Study the drawing (mm; zero at the part's minimum x, y, z) and answer. A direction names the side the tool comes from. Coordinates: 2 decimals unless noted, no trailing zeros. Loops run counter-clockwise (first coordinate to the right, second up) from the corner with the lowest first, then second, coordinate; pieces in that order, holes last. Notation, with made-up numbers: (51, 42.5) -> (70, 42.5) arc R25 cw to (70, 57.5) -> close; hole circle Ø2 at (16, -21). An arc over 180 degrees is marked (long way). Answer as a JSON object with one key per item and string values. Group by question number.
Q1. The part is cut by section A-A on x = 27.5. Write down the section's boundary in (y, z), and give its area (3 significant figures).
Q2. For the marked faces 1, 2 and 3, determine the directions among +Z, -Z, +X, -X, +Y, -Y from which every point of the face is accessible in a straight line to the end or side of a thin tool.
Q3. Each of these flat-tipped pins is pushed along its axis until it touches: P1, Ø1, axis at y = 12.5, z = 3.5, coming from the -X side; P2, Ø13, axis at x = 7, y = 17, coming from the -Z side; P3, Ø1, axis at x = 17, y = 24.5, coming from the +Z side. Where does it stop, or does it pass through?
Q4. Determine the mould class of the marked faces 4, 5 and 6 for opening direction X: released by +X, released by -X, zero draft, split by the parting line, or undercut.
Q5. The part is cut by section B-B on y = 11.5. State how many separate pieces and enclosed holes the cut face has, and give its area (3 significant figures).
Q6. Straight lines are drawn through the part: line 1 along X through (y, z) = (11.4, 2.5); line 2 along Y through (x, z) = (15.25, 2); line 3 along X through (y, z) = (11.75, 3.3). For each, find the intervals that lie inside material, in ascending order. Write a range as [from, to].
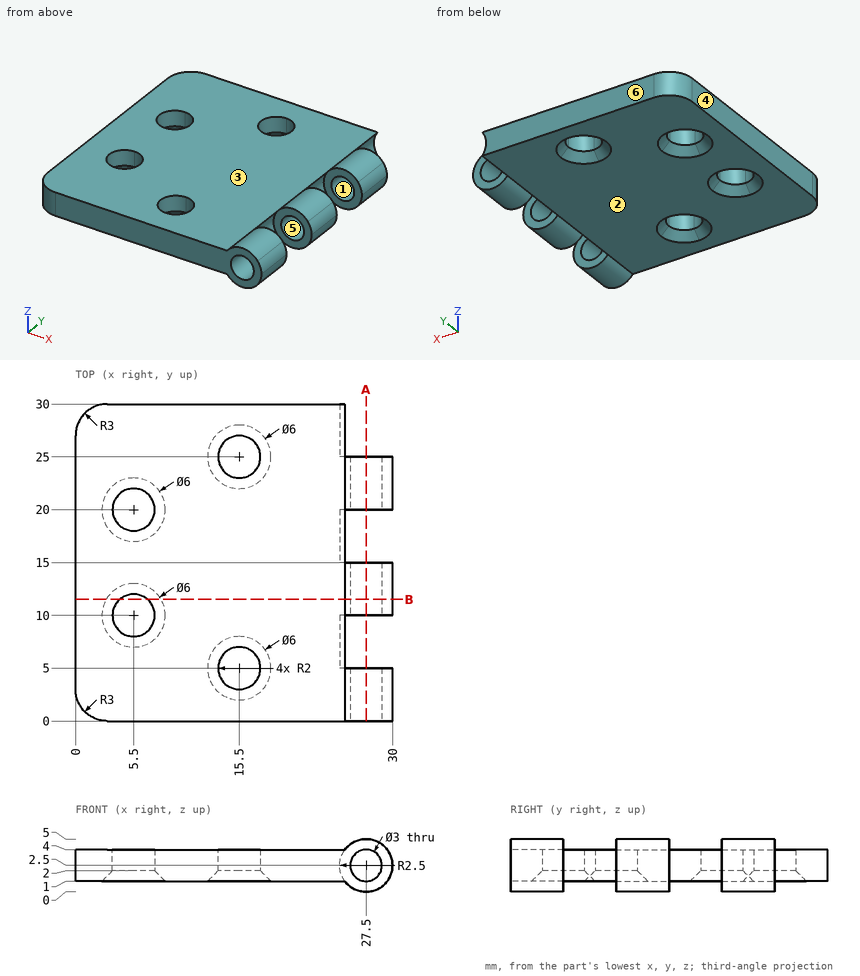
Final values:
{
 "1": {"outline": "(0, 0) -> (5, 0) -> (5, 1) -> (0, 1) -> close; (0, 4) -> (5, 4) -> (5, 5) -> (0, 5) -> close; (10, 0) -> (15, 0) -> (15, 1) -> (10, 1) -> close; (10, 4) -> (15, 4) -> (15, 5) -> (10, 5) -> close; (20, 0) -> (25, 0) -> (25, 1) -> (20, 1) -> close; (20, 4) -> (25, 4) -> (25, 5) -> (20, 5) -> close", "area": "30.0 mm2"},
 "2": {"face 1": "+Y, -Y", "face 2": "-Z, -X, +Y, -Y", "face 3": "+Z, -X, +Y, -Y"},
 "3": {"P1": "stops at x = 0", "P2": "stops at z = 1", "P3": "stops at z = 4"},
 "4": {"face 4": "released by -X", "face 5": "undercut", "face 6": "zero draft"},
 "5": {"separate pieces": "2", "enclosed holes": "1", "area": "78.8 mm2"},
 "6": {"line 1": "x = [0, 4.07], [6.93, 26], [29, 30]", "line 2": "y = [0, 3.02], [6.98, 23.02], [26.98, 30]", "line 3": "x = [0, 4.53], [6.47, 26.23], [28.77, 29.87]"}
}
